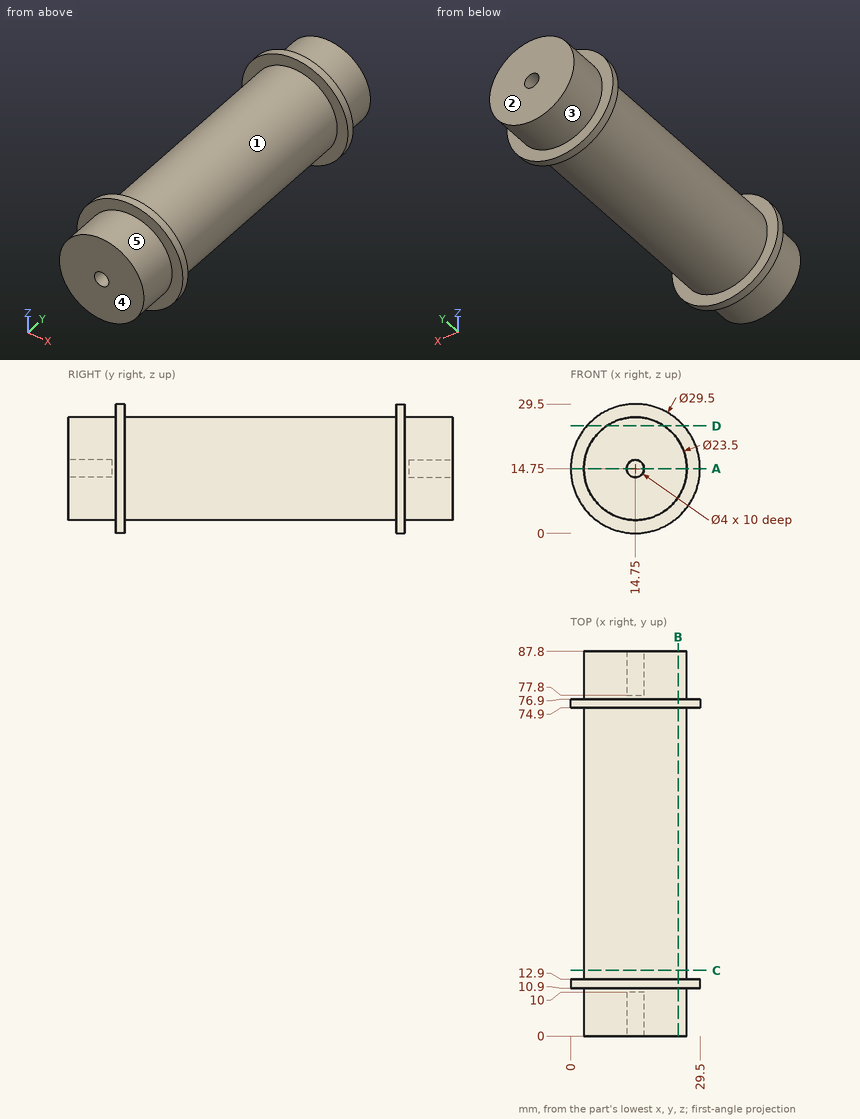
Geometry: see drawing. Coordinates: mm, zero at the bounding-box minimum. A direction names the side the tool comes from. Round coordinates to 2 decimals unless told otherwise and drop trailing zeros. Loops run counter-clockwise (first coordinate to the right, second up) from the corner with the lowest first, then second, coordinate; pieces in that order, holes last. Notation, with made-up numbers: M 22.5,84.25 L 45.5,84.25 A14 ccw 45.5,96.25 Z; hole C 4.5,8 d1. An arc over 180 degrees is marked long. Use a Markdown table: item, result. Add a question column.
1. Reachability of the marked faces 4 and 5 from +Z, -Z, +X, -X, +Y, -Y: full face, straight path, thin tool, end or side. Return the list, or none.
2. Mould query, pull axis Y, two halves, no side actions, for the marked faces 1, 2 and 3. Classes: pulls with the +Y half, pulls with the -Y half, needs draft (parallel to the pull), parting line crosses it, or undercut.
3. Section query B-B on x = 24.5. Return the cut outline in (y, z), then the cut area to 3 significant figures.
4. Contact query for flat-ended pins moving along their axis: P1, Ø5, axis at y = 50, z = 25, coming from the -X side; P2, Ø3, axis at x = 14, z = 14.5, coming from the -Y side; P3, Ø3, axis at y = 48, z = 5, coming from the +X side; P4, Ø3.5, axis at x = 14.75, z = 14.75, coming from the -Y side. Output: stop coordinate, or through.
5. Section query A-A on z = 14.75. Return the cut outline in (x, y).
6. Section query D-D on z = 24.5. Return the cut outline in (x, y).
7. Line query: line 1 (Z direction, x = 14.75, y = 81.5); line 2 (Y direction, x = 25, z = 22); line 3 (X direction, y = 30, z = 14.5). Output: solid intervals per line, ascending.
8. Section query C-C on y = 15. Return the cut outline in (x, z).
Reported:
| question | item | result |
|---|---|---|
| 1 | face 4 | +Z, -Z, +X, -X, -Y |
| 1 | face 5 | -Y |
| 2 | face 1 | undercut |
| 2 | face 2 | pulls with the +Y half |
| 2 | face 3 | needs draft |
| 3 | outline | M 0,8.19 L 10.9,8.19 L 10.9,3.68 L 12.9,3.68 L 12.9,8.19 L 74.9,8.19 L 74.9,3.68 L 76.9,3.68 L 76.9,8.19 L 87.8,8.19 L 87.8,21.31 L 76.9,21.31 L 76.9,25.82 L 74.9,25.82 L 74.9,21.31 L 12.9,21.31 L 12.9,25.82 L 10.9,25.82 L 10.9,21.31 L 0,21.31 Z |
| 3 | area | 1,190 mm² |
| 4 | P1 | stops at x = 5.92 |
| 4 | P2 | stops at y = 0 |
| 4 | P3 | stops at x = 23.12 |
| 4 | P4 | stops at y = 10 |
| 5 | outline | M 0,10.9 L 3,10.9 L 3,0 L 12.75,0 L 12.75,10 L 16.75,10 L 16.75,0 L 26.5,0 L 26.5,10.9 L 29.5,10.9 L 29.5,12.9 L 26.5,12.9 L 26.5,74.9 L 29.5,74.9 L 29.5,76.9 L 26.5,76.9 L 26.5,87.8 L 16.75,87.8 L 16.75,77.8 L 12.75,77.8 L 12.75,87.8 L 3,87.8 L 3,76.9 L 0,76.9 L 0,74.9 L 3,74.9 L 3,12.9 L 0,12.9 Z |
| 6 | outline | M 3.68,10.9 L 8.19,10.9 L 8.19,0 L 21.31,0 L 21.31,10.9 L 25.82,10.9 L 25.82,12.9 L 21.31,12.9 L 21.31,74.9 L 25.82,74.9 L 25.82,76.9 L 21.31,76.9 L 21.31,87.8 L 8.19,87.8 L 8.19,76.9 L 3.68,76.9 L 3.68,74.9 L 8.19,74.9 L 8.19,12.9 L 3.68,12.9 Z |
| 7 | line 1 | z = 3 to 12.75, 16.75 to 26.5 |
| 7 | line 2 | y = 10.9 to 12.9, 74.9 to 76.9 |
| 7 | line 3 | x = 3 to 26.5 |
| 8 | outline | C 14.75,14.75 d23.5 |
